CAD build for the part. Positions are in the model's coordinates, mm. Face numbers are marked on the shaded views. Coordinates: 2 decimals unless noted, no trailing zeros. Loops run counter-clockwise (first coordinate to the right, second up) from the corner with the lowest first, then second, coordinate; pieces in that order, holes last. Notation, with made-up numbers: (-26, -4.75) -> (-2, -4.75) arc R29 ccw to (-2, 25.25) -> close; hole circle Ø7 at (0.5, 8). An arc over 180 degrees is marked (long way). Return JSON: item names as keys, results as strings. Group by question number.
(1) Saw through at B-B on y = -34. Write the cut outline in (x, z).
(2) Flat gauge pins, fed straight in: pin 1 Ø11.5 at (x, y) = (18.66, 25.69) entering from -Z; pin 2 Ø1.5 at (x, z) = (8, 17) entering from -Y; pin 3 Ø12 at (x, z) = (5, 2.5) entering from +Y; pin 4 Ø4 at (x, z) = (1.5, 11.5) entering from -Y. Where does each tip first touch, or does it go through?
(3) Saw through at C-C on z = 22.25. Write the cut outline in (x, y).
(4) Probe L1, parallel to Y at x = 16.5, z = 22.5; L2, parallel to Y at x = 26.5, z = 5; L3, parallel to X at y = -34, z = 23.25. List the from-to ranges inside material, lowest first.
(5) Saw through at D-D on y = 18. Write the cut outline in (x, z).
(6) Saw through at A-A on x = 0. Write the cut outline in (y, z), then the cut area to 3 significant figures.
(7) Mould opens along X. For the marked faces 1, 2 and 3 say: pulls with the +X half, pulls with the -X half, needs draft (parallel to the pull), parting line crosses it, or undercut.
```python
from build123d import *

# Parameters (mm, degrees)
F0_R            = 50.8
F1_DEPTH        = 25.4
F2_R            = 6.35
F4_DEPTH        = 25.401
F4_COPIES_COUNT = 5


# Not quite as in the source:
# - a pattern or mirror of a feature is missing from the dataset's text; its kind, count and spacing are read off the source's solid


with BuildPart() as f1:
    # F0 (on Top) → F1 (new body)
    with BuildSketch(Plane.XY):
        Circle(F0_R)
    extrude(amount=F1_DEPTH)

    # F2 (on face) → F4 (cut, through all)
    with BuildSketch(Plane.XY.offset(25.4)):
        with Locations((0, -31.75)):
            Circle(F2_R)
    f4 = extrude(amount=-F4_DEPTH, mode=Mode.SUBTRACT)

    # F4_copies: F4 ×5 about axis
    f4_copies_axis = Axis((0, 0, 0), (0, 0, 1))
    for i in range(1, F4_COPIES_COUNT):
        add(f4.rotate(f4_copies_axis, i * 360 / F4_COPIES_COUNT), mode=Mode.SUBTRACT)


solid = f1.part
```
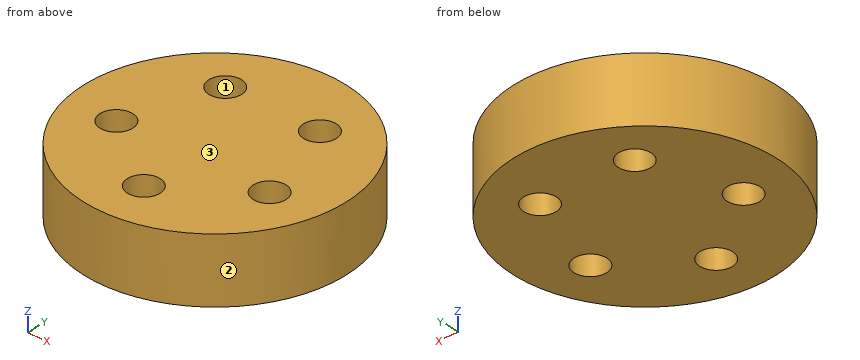
Geometry results:
{
 "1": {"outline": "(-37.74, 0) -> (-5.94, 0) -> (-5.94, 25.4) -> (-37.74, 25.4) -> close; (5.94, 0) -> (37.74, 0) -> (37.74, 25.4) -> (5.94, 25.4) -> close"},
 "2": {"pin 1": "through", "pin 2": "y = -50.28", "pin 3": "y = 50.8", "pin 4": "y = -50.8"},
 "3": {"outline": "circle Ø101.6 at (0, 0); hole circle Ø12.7 at (-30.2, -9.81); hole circle Ø12.7 at (-18.66, 25.69); hole circle Ø12.7 at (0, -31.75); hole circle Ø12.7 at (18.66, 25.69); hole circle Ø12.7 at (30.2, -9.81)"},
 "4": {"L1": "-48.05 to 19.72, 31.66 to 48.05", "L2": "-43.34 to -14.97, -4.65 to 43.34", "L3": "-37.74 to -5.94, 5.94 to 37.74"},
 "5": {"outline": "(-47.5, 0) -> (47.5, 0) -> (47.5, 25.4) -> (-47.5, 25.4) -> close"},
 "6": {"outline": "(-50.8, 0) -> (-38.1, 0) -> (-38.1, 25.4) -> (-50.8, 25.4) -> close; (-25.4, 0) -> (50.8, 0) -> (50.8, 25.4) -> (-25.4, 25.4) -> close", "area": "2,260 mm²"},
 "7": {"face 1": "undercut", "face 2": "parting line crosses it", "face 3": "needs draft"}
}
